```python
from build123d import *

# Parameters (mm, degrees)
SKETCH1_W           = 90
SKETCH1_H           = 46
SKETCH1_W_2         = 41
SKETCH1_H_2         = 22
BOSS_EXTRUDE1_DEPTH = 6
BOSS_EXTRUDE2_DEPTH = 26


with BuildPart() as part:
    # Sketch1 → Boss-Extrude1 (new body)
    with BuildSketch(Plane(origin=(0, 0, 0), x_dir=(1, 0, 0), z_dir=(0, 1, 0))):
        with Locations((45, 23)):
            Rectangle(SKETCH1_W, SKETCH1_H)
        with Locations((49.5, 27)):
            Rectangle(SKETCH1_W_2, SKETCH1_H_2, mode=Mode.SUBTRACT)
    extrude(amount=BOSS_EXTRUDE1_DEPTH)

    # Sketch2 → Boss-Extrude2 (add)
    with BuildSketch(Plane.XZ):
        Polygon((0, 0), (4, 0), (82, 0), (90, 0), (90, -30), (86, -30), (86, -2), (4, -2), (4, -30), (0, -30), align=None)
        Polygon((37.5, -46), (52.5, -46), (45, -38), align=None)
    extrude(amount=BOSS_EXTRUDE2_DEPTH)


solid = part.part
```
Model file for the job. Use its own axes, mm. A direction names the side the tool comes from. Give positions to 0.01 mm unless a question says otherwise; leave off trailing zeros. Write each loop counter-clockwise with the first axis right and the second up, starting at its lowest first coordinate (ties: lowest second). Pieces come first, ordered by that corner, then holes. Notation, with made-up numbers: (13.5, 59.5) -> (32.5, 59.5) arc R7 cw to (32.5, 65.5) -> close; hole circle Ø5 at (45.5, 58.25). An arc over 180 degrees is marked (long way). Use CSV: the item, a comma, the result in double quotes. Start each with the question number.
1) Cut at B-B on y = -17. List the corners of the cut face in (x, z), plus the area to 3 significant figures.
2) Cut at D-D on z = -13. List the corners of the cut face in (x, y), plus the area to 3 significant figures.
3) Pin check, flat tips, straight feed: P1, Ø2, axis at x = 10, z = -33.5, coming from the -Y side; P2, Ø3, axis at x = 2, y = -18, coming from the -Z side. Stop position of each tip, or through.
4) Cut at C-C on x = 31. List the corners of the cut face in (y, z).
5) Two-plate mould, pull along Z, no slides. Class faces 1 (the flat face through (29, 3, -27)), 2 (the flat face through (86, -13, -16)), 3 (the flat face through (45, -4, -46)): released by +Z, released by -Z, zero draft, split by the parting line, or undercut.
6) Drill centre lines: L1, parallel to X at y = -3.5, z = -12; L2, parallel to Y at x = 48, z = -6; L3, parallel to Z at x = 10, y = -24. Where is each one in solid material? Low to high.
7) Tool access for faces 4 (the flat face through (49, 3, -38)), 5 (the flat face through (4, -13, -16)), 6 (the flat face through (48.802, -12.818, -42.056)), 7 (the flat face through (2, -13, -30)): list every direction of +Z, -Z, +X, -X, +Y, -Y with a clear straight run to the whole face (end or side of a thin tool).
8) Cut at A-A on z = -23. List the corners of the cut face in (x, y), plus the area to 3 significant figures.
Final values:
1,outline,"(0, -30) -> (4, -30) -> (4, -2) -> (86, -2) -> (86, -30) -> (90, -30) -> (90, 0) -> (0, 0) -> close; (37.5, -46) -> (52.5, -46) -> (45, -38) -> close"
1,area,"464 mm2"
2,outline,"(0, -26) -> (4, -26) -> (4, 0) -> (86, 0) -> (86, -26) -> (90, -26) -> (90, 6) -> (0, 6) -> close"
2,area,"748 mm2"
3,P1,"stops at y = 0"
3,P2,"stops at z = -30"
4,outline,"(-26, -2) -> (0, -2) -> (0, -16) -> (6, -16) -> (6, 0) -> (-26, 0) -> close; (0, -46) -> (6, -46) -> (6, -38) -> (0, -38) -> close"
5,face 1,"undercut"
5,face 2,"zero draft"
5,face 3,"released by -Z"
6,L1,"x = 0 to 4, 86 to 90"
6,L2,"y = 0 to 6"
6,L3,"z = -2 to 0"
7,face 4,"+Y, -Y"
7,face 5,"-Z, -Y"
7,face 6,"+X, -Y"
7,face 7,"-Z, +X, -X, -Y"
8,outline,"(0, -26) -> (4, -26) -> (4, 0) -> (29, 0) -> (29, 6) -> (0, 6) -> close; (70, 0) -> (86, 0) -> (86, -26) -> (90, -26) -> (90, 6) -> (70, 6) -> close"
8,area,"502 mm2"
